Read the model definition and answer for the solid it produces. Units are mm, in the model's axes. Face numbers are marked on the shaded views. A direction names the side the tool comes from. Coordinates: 2 decimals unless noted, no trailing zeros. Write each loop counter-clockwise with the first axis right and the second up, starting at its lowest first coordinate (ties: lowest second). Pieces come first, ordered by that corner, then holes. Notation, with made-up numbers: (5.5, 29) -> (61.5, 29) arc R31 ccw to (61.5, 56) -> close; hole circle Ø4 at (34, 42.5). An arc over 180 degrees is marked (long way). One line per item, written item: value. Start each with the question number.
1. Find section D-D, the plane z = 2.5. Write down the section's boundary in (x, y).
2. Given P1, Ø0.8, axis at x = 2.5, z = -1.5, coming from the -Y side; P2, Ø2, axis at x = 0.5, y = 1.5, coming from the -Z side; P3, Ø3, axis at y = -16.5, z = 0.5, coming from the +X side, each flat-ended and moving along its own axis, determine where each tip first touches the part or whether it passes through.
3. Find section C-C, the plane y = 0.5. Write down the section's boundary in (x, z).
4. Find section B-B, the plane z = -4. Write down the section's boundary in (x, y).
5. For the marked faces 1, 2, 3 and 4, determine the directions among +Z, -Z, +X, -X, +Y, -Y from which every point of the face is accessible in a straight line to the end or side of a thin tool.
6. Find section A-A, the plane x = 1. Write down the section's boundary in (y, z), and give its area (3 significant figures).
7. Consider line 1 along Y through (x, z) = (3.25, -3); line 2 along X through (y, z) = (-9, -0.5); line 3 along Z through (x, y) = (1, 2.5). Determine where each line is inside the solid, lowest interval first.
Autodesk Inventor part; units mm, degrees
ref_plane "YZ Plane" through (0, 0, 0) normal (1, 0, 0) x (0, 1, 0)
ref_plane "XZ Plane" through (0, 0, 0) normal (0, 1, 0) x (-1, 0, 0)
ref_plane "XY Plane" through (0, 0, 0) normal (0, 0, 1) x (1, 0, 0)
sketch "Sketch1" plane through (0, 0, 0) normal (0, 1, 0) x (-1, 0, 0)
  line L0 (-1.8, -4.8) -> (1.8, -4.8)
  line L1 (1.8, -4.8) -> (1.8, 4.8)
  line L2 (1.8, 4.8) -> (-1.8, 4.8)
  line L3 (-1.8, 4.8) -> (-1.8, -4.8)
  line L4 (-1.8, -4.8) -> (1.8, 4.8) construction
  line L5 (1.8, -4.8) -> (-1.8, 4.8) construction
  point P0 (0, 0)
  dimension "d0" = 3.6
  dimension "d1" = 9.6
extrude "Extrusion1" add sketch "Sketch1" along normal blind 8
sketch "Sketch2" plane through (0, 0, 0) normal (0, -1, 0) x (1, 0, 0)
  line L0 (-4, -5) -> (4, -5)
  line L1 (4, -5) -> (4, 5)
  line L2 (4, 5) -> (-4, 5)
  line L3 (-4, 5) -> (-4, -5)
  line L4 (-4, -5) -> (4, 5) construction
  line L5 (4, -5) -> (-4, 5) construction
  point P0 (0, 0)
  dimension "d4" = 8
  dimension "d5" = 10
extrude "Extrusion2" add sketch "Sketch2" along normal blind 23
fillet "Fillet1" radius 7 1 edges at (0, -23, 5)
sketch "Sketch3" plane through (4, 0, -5) normal (0, 0, -1) x (-1, 0, 0)
  line L0 (0, 0) -> (0, -16)
  line L1 (8, -23) -> (0, -23)
  line L2 (0, -3) -> (0, -23)
  line L3 (0, -23) -> (2.5, -23)
  line L4 (2.5, -23) -> (2.5, -3)
  line L5 (2.5, -3) -> (0, -3)
  line L6 (8, 0) -> (0, 0)
  line L7 (4, 0) -> (4, -23) construction
  line L8 (8, -3) -> (8, -23)
  line L9 (8, -23) -> (5.5, -23)
  line L10 (5.5, -23) -> (5.5, -3)
  line L11 (5.5, -3) -> (8, -3)
  point P0 (8, -16)
  dimension "d9" = 1.5
  dimension "d10" = 3
extrude "Extrusion3" cut sketch "Sketch3" against normal up to next
sketch "Sketch4" plane through (0, 8, 0) normal (0, 1, 0) x (1, 0, 0)
  line L0 (2, 5) -> (-2, 5)
  line L1 (-2, 5) -> (-2, -5)
  line L2 (-2, -5) -> (2, -5)
  line L3 (2, -5) -> (2, 5)
  line L4 (2, 5) -> (-2, -5) construction
  line L5 (-2, 5) -> (2, -5) construction
  point P0 (0, 0)
  dimension "d13" = 4
  dimension "d14" = 10
properties part number "lavalier_holder"
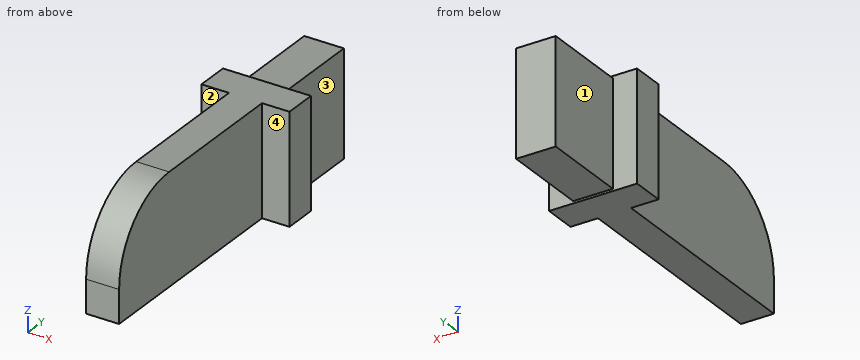
Answer block:
1. outline: (-4, -3) -> (-1.5, -3) -> (-1.5, -21.36) -> (1.5, -21.36) -> (1.5, -3) -> (4, -3) -> (4, 0) -> (1.8, 0) -> (1.8, 8) -> (-1.8, 8) -> (-1.8, 0) -> (-4, 0) -> close
2. P1: stops at y = -3
2. P2: stops at z = -4.8
2. P3: stops at x = 1.5
3. outline: (-1.8, -4.8) -> (1.8, -4.8) -> (1.8, 4.8) -> (-1.8, 4.8) -> close
4. outline: (-4, -3) -> (-1.5, -3) -> (-1.5, -23) -> (1.5, -23) -> (1.5, -3) -> (4, -3) -> (4, 0) -> (1.8, 0) -> (1.8, 8) -> (-1.8, 8) -> (-1.8, 0) -> (-4, 0) -> close
5. face 1: +Z, -Z, -X, +Y
5. face 2: +Z, -Z, -X, -Y
5. face 3: +Z, -Z, +X, +Y
5. face 4: +Z, -Z, +X, -Y
6. outline: (-23, -5) -> (0, -5) -> (0, -4.8) -> (8, -4.8) -> (8, 4.8) -> (0, 4.8) -> (0, 5) -> (-16, 5) arc R7 ccw to (-23, -2) -> close
6. area: 296 mm2
7. line 1: y = -3 to 0
7. line 2: x = -1.5 to 1.5
7. line 3: z = -4.8 to 4.8
